CAD build for the part. Positions are in the model's coordinates, mm. A direction names the side the tool comes from. Round coordinates to 2 decimals unless told otherwise and drop trailing zeros. Write each loop counter-clockwise with the first axis right and the second up, starting at its lowest first coordinate (ties: lowest second). Pieces come first, ordered by that corner, then holes. Notation, with made-up numbers: M 7,18 L 49,18 A13 cw 49,38 Z; hole C -34.5,-0.75 d1. An arc over 180 degrees is marked long. Write each question's results on one line, items separated by ' | '. Start each with the question number.
Autodesk Fusion 360 part; units mm, degrees
sketch "Sketch1" plane through (0, 0, 0) normal (0, 0, 1) x (1, 0, 0)
  line L0 (35, 45) -> (-35, 45)
  line L1 (-35, 45) -> (-35, -45)
  line L2 (-35, -45) -> (35, -45)
  line L3 (35, -45) -> (35, 45)
  line L4 (35, 45) -> (-35, -45) construction
  line L5 (-35, 45) -> (35, -45) construction
  line L6 (0, 28.3109) -> (0, -26.5165) construction
  line L7 (-6.5, 15) -> (-6.5, -16.8183) construction
  dimension "d1" = 70
  dimension "d2" = 90
  dimension "d3" = 6.5
extrude "Extrude1" add sketch "Sketch1" along normal blind 3 makes body 1
sketch "Sketch2" plane through (0, 0, 3) normal (0, 0, 1) x (-1, 0, 0)
  line L0 (-35, 45) -> (-35, -45)
  line L1 (-35, -45) -> (35, -45)
  line L2 (35, -45) -> (35, 45)
  line L3 (35, 45) -> (-35, 45)
  line L4 (6.5, 18.4092) -> (11, 18.4092)
  line L5 (11, 18.4092) -> (11, -16.5908)
  line L6 (11, -16.5908) -> (6.5, -16.5908)
  line L7 (6.5, -16.5908) -> (6.5, 18.4092)
  line L8 (6.5, -15) -> (6.5, 16.8183)
  dimension "d6" = 4.5
  dimension "d7" = 35
extrude "Extrude2" add sketch "Sketch2" along normal blind 35 contours L4 L5 L6 L7 L8 bodies 1
sketch "Sketch3" plane through (0, 0, 3) normal (0, 0, 1) x (-1, 0, 0)
  line L0 (6.5, 18.4092) -> (11, 18.4092)
  line L1 (11, 18.4092) -> (11, -16.5908)
  line L2 (11, -16.5908) -> (6.5, -16.5908)
  line L3 (6.5, -16.5908) -> (6.5, 18.4092)
  line L4 (-35, 45) -> (-35, -45)
  line L5 (-35, -45) -> (35, -45)
  line L6 (35, -45) -> (35, 45)
  line L7 (35, 45) -> (-35, 45)
  line L8 (34, 44) -> (-34, 44)
  line L9 (-34, 44) -> (-34, -44)
  line L10 (-34, -44) -> (34, -44)
  line L11 (34, -44) -> (34, 44)
  line L12 (34, 44) -> (-34, -44) construction
  line L13 (-34, 44) -> (34, -44) construction
  dimension "d10" = 68
  dimension "d11" = 88
extrude "Extrude3" add sketch "Sketch3" along normal blind 10 contours L4 L5 L6 L7 bodies 1
sketch "Sketch4" plane through (-11, 0, 0) normal (-1, 0, 0) x (0, -1, 0)
  line L0 (-16.5908, 3) -> (18.4092, 3)
  line L1 (18.4092, 3) -> (18.4092, 38)
  line L2 (18.4092, 38) -> (-16.5908, 38)
  line L3 (-16.5908, 38) -> (-16.5908, 3)
  circle A0 centre (0.9092, 20.5) radius 8.8
  line L4 (-16.5908, 3) -> (-16.5908, 38)
  line L5 (-16.5908, 38) -> (18.4092, 38)
  line L6 (18.4092, 3) -> (18.4092, 38)
  line L7 (18.4092, 3) -> (-16.5908, 3)
  line L8 (-16.5908, 38) -> (18.4092, 3) construction
  line L9 (10.9092, 3) -> (13.7611, 3)
  line L10 (13.7611, 3) -> (13.7611, 19.5)
  line L11 (12.7611, 20.5) -> (11.9092, 20.5)
  line L12 (10.9092, 19.5) -> (10.9092, 3)
  line L13 (-5.4652, 20.5) -> (30.4752, 20.5) construction
  arc A1 (11.9092, 20.5) -> (10.9092, 19.5) centre (11.9092, 19.5) ccw
  arc A2 (13.7611, 19.5) -> (12.7611, 20.5) centre (12.7611, 19.5) ccw
  dimension "d14" = 17.6
  dimension "d15" = 10
  dimension "d16" = 1
extrude "Extrude4" add sketch "Sketch4" along normal blind 4 separate body contours L0 L7 L9 L10 L11 L12 A1 A2 makes body 2
move_body "Move1" bodies 2 to x (1, 0, 0) y (0, 1, 0) z (0, 0, 1) at (-13, 0, 0)
sketch "Sketch5" plane through (-28, 0, 0) normal (-1, 0, 0) x (0, -1, 0)
  arc A0 (13.7611, 19.5) -> (12.7611, 20.5) centre (12.7611, 19.5) ccw
  line L0 (12.7611, 20.5) -> (11.9092, 20.5)
  arc A1 (11.9092, 20.5) -> (10.9092, 19.5) centre (11.9092, 19.5) ccw
  line L1 (10.9092, 19.5) -> (10.9092, 3)
  line L2 (10.9092, 3) -> (13.7611, 3)
  line L3 (13.7611, 3) -> (13.7611, 19.5)
  line L4 (13.7611, 19.5) -> (23.2874, 3)
  line L5 (13.7611, 19.5) -> (32.9491, 19.5) construction
  line L6 (23.2874, 3) -> (10.9092, 3)
  line L7 (13.7611, 19.5) -> (13.7611, 3)
  line L8 (15.7611, 12.0359) -> (21.5554, 2)
  line L9 (15.7611, 12.0359) -> (15.7611, 3)
  dimension "d19" = 60
  dimension "d20" = -2
extrude "Extrude5" add sketch "Sketch5" against normal blind 4 contours L3 L4 L6 L7 L8 L9 bodies 1 2
extrude "Extrude6" cut sketch "Sketch4" against normal blind 6 contours A0 bodies 1
1) Wall check: line 1 along Y through (x, z) = (14, 4); line 2 along X through (y, z) = (33.5, 7.5); line 3 along Y through (x, z) = (-8, 20). Give the ranges that are in metal, low to high. Write a range as from..to.
2) 3-axis set-ups, long thin cutter, end or side, ignore diameter. For faces 1 (the face through (-26, -15.761, 8)), 2 (the face through (-34, 1, 8)), 3 (the face through (0, -45, 6)): which of +Z, -Z, +X, -X, +Y, -Y reach the whole face in a straight line?
3) Saw through at D-D, the plane x = -22.5. Write the cut outline in (y, z).
4) Pull direction Y, two halves, no side cores. Call faces 4 (the face through (0, 45, 6)), 5 (the face through (-11, -5, 12)), 6 (the face through (35, -1, 6)): pulls with the +Y half, pulls with the -Y half, needs draft (parallel to the pull), parting line crosses it, or undercut.
5) Drop flat-ended pins along their axis: pin 1 Ø1.3 at (x, z) = (-9.5, 25.5) entering from +Y; pin 2 Ø5 at (x, z) = (-8, 27.5) entering from -Y; pin 3 Ø5 at (y, z) = (1, 32) entering from +X. Give the stop position or say it passes through.
6) Saw through at B-B, the plane y = 20.5. Write the cut outline in (x, z).
7) Saw through at A-A, the plane z = 8. Write the cut outline in (x, y), plus the area to 3 significant figures.
8) Saw through at C-C, the plane y = -1.5. Write the cut outline in (x, z).
Filled sheet:
1) line 1: y = -45..-44, 44..45 | line 2: x = -35..-34, 34..35 | line 3: y = -18.41..-9.69, 7.88..16.59
2) face 1: none | face 2: +Z | face 3: +Z, -Z, +X, -X, -Y
3) outline: M -45,0 L 45,0 L 45,13 L 44,13 L 44,3 L -44,3 L -44,13 L -45,13 Z
4) face 4: pulls with the +Y half | face 5: undercut | face 6: needs draft
5) pin 1: stops at y = 16.59 | pin 2: stops at y = -18.41 | pin 3: stops at x = -6.5
6) outline: M -35,0 L 35,0 L 35,13 L 34,13 L 34,3 L -34,3 L -34,13 L -35,13 Z
7) outline: M -35,-45 L 35,-45 L 35,45 L -35,45 Z; M -28,-20.4 L -24,-20.4 L -24,-18.09 L -28,-18.09 Z; M -28,-15.76 L -24,-15.76 L -24,-10.91 L -28,-10.91 Z; M -11,-18.41 L -6.5,-18.41 L -6.5,16.59 L -11,16.59 Z; hole M -34,-44 L 34,-44 L 34,44 L -34,44 Z | area: 502 mm^2
8) outline: M -35,0 L 35,0 L 35,13 L 34,13 L 34,3 L -6.5,3 L -6.5,11.72 L -11,11.72 L -11,3 L -34,3 L -34,13 L -35,13 Z; M -11,29.28 L -6.5,29.28 L -6.5,38 L -11,38 Z
